Design review of the part built by this model. Coordinates are the model's own, in mm. A direction names the side the tool comes from. Give positions to 0.01 mm unless a question says otherwise; leave off trailing zeros. Order: outer loops, then holes, each group sorted by start corner. A loop starts at its lowest first (then second) coordinate and runs counter-clockwise, first axis right, second up. Notation, with made-up numbers: M -22.75,34 L -13.75,34 A36 ccw -13.75,70 Z; hole C -17.5,9 d4. An arc over 180 degrees is marked long. Answer as a JSON object with one key per item and string values.
Autodesk Inventor part; units mm, degrees
ref_plane "Work Plane1" through (1.525, 0, 0) normal (0, 0, 1) x (1, 0, 0)
ref_plane "YZ Plane" through (0, 0, 0) normal (1, 0, 0) x (0, 1, 0)
ref_plane "XZ Plane" through (0, 0, 0) normal (0, 1, 0) x (-1, 0, 0)
sketch "Sketch1" plane through (0, 0, 0) normal (0, 0, 1) x (1, 0, 0)
  line L0 (0, 5.0006) -> (0, 3.175)
  line L1 (3.175, 3.175) -> (22.225, 3.175)
  line L2 (22.225, 3.175) -> (22.225, 0)
  line L3 (22.225, 0) -> (-0.6351, 0)
  line L4 (-5.2071, 0) -> (26.797, 0)
  line L5 (-0.6351, 0) -> (-0.6351, 5.0006)
  line L6 (-0.6351, 5.0006) -> (0, 5.0006)
  line L7 (3.175, 3.175) -> (1.9049, 3.175)
  line L8 (1.9049, 3.175) -> (0, 3.175)
  line L9 (0, -1.0001) -> (0, 6.0007)
  dimension "d0" = 22.225
  dimension "d1" = 19.05
  dimension "d2" = 6.35
  dimension "d9" = 0.6351
  dimension "d10" = 10.0013
  dimension "d13" = 1.2701
  dimension "d14" = 6.35
revolve "Body" add sketch "Sketch1" angle 360 about axis through (22.225, 0, 0) along (-1, 0, 0)
sketch "Sketch2" plane through (-0.6351, 0, 0) normal (-1, 0, 0) x (0, 0, 1)
  line L0 (0, 6.4158) -> (5.5562, 3.2079)
  line L1 (5.5562, 3.2079) -> (5.5562, -3.2079)
  line L2 (5.5562, -3.2079) -> (0, -6.4158)
  line L3 (0, -6.4158) -> (-5.5562, -3.2079)
  line L4 (-5.5562, -3.2079) -> (-5.5562, 3.2079)
  line L5 (-5.5562, 3.2079) -> (0, 6.4158)
  point P0 (0, 0)
  point P1 (0, 0)
  dimension "d11" = 11.1125
extrude "Head" add sketch "Sketch2" along normal blind 3.3337
sketch "Sketch4" plane through (0, 0, 0) normal (0, 0, 1) x (1, 0, 0)
  line L0 (-3.9689, 5.5563) -> (-3.9689, 6.4158)
  line L1 (-3.9689, 6.4158) -> (-3.4726, 6.4158)
  line L2 (-3.4726, 6.4158) -> (-3.9689, 5.5563)
  line L3 (-4.6356, 0) -> (0.0317, 0)
  line L4 (-0.6351, 6.4158) -> (-3.9688, 6.4158)
  line L5 (-3.9688, 3.2079) -> (-3.9688, 6.4158)
  dimension "d5" = 30
  dimension "d19" = 11.1125
revolve "Chamfer1" cut sketch "Sketch4" angle 360 about axis through (-10, 0, 0) along (1, 0, 0)
thread "Thread"
chamfer "Chamfer2" distance 0.6875 distance2 1.2701 1 edges at (22.225, -3.175, 0) measured on face at (22.225, -0.1276, -1.0506)
ref_plane "Work Plane1" through (1.525, 0, 0) normal (0, 0, 1) x (1, 0, 0)
fillet "Fillet2" radius 0.635 1 edges at (0, -3.175, 0)
equation "\"d0\" = NLG"
equation "\"d1\" = GEL"
equation "\"d2\" = GD"
equation "\"d10\" = SD2"
equation "\"d14\" = BDM"
equation "\"d11\" = SW"
equation "\"d3\" = KOH - SD"
equation "\"d5\" = ANG1"
equation "\"d19\" = SW0"
equation "\"d63\" = R"
equation "\"d15\" = GEL"
equation "\"d6\" = -0.5 * SPD + 0.5 * GD"
equation "\"NLG\" = 22.225"
equation "\"GD\" = NND"
equation "\"BDM\" = 6.35"
equation "\"KOH\" = 3.96875"
equation "\"GEL\" = 19.05"
equation "\"SW\" = 11.1125"
equation "\"SW0\" = SW"
equation "\"SPD\" = 4.9751"
equation "\"SD2\" = 10.00125"
equation "\"SD\" = 0.635"
equation "\"ANG1\" = 30deg"
equation "\"GAL\" = 1.27"
equation "\"GUL\" = 1.27"
equation "\"R\" = 0.635"
equation "\"d62\" = -NLG - SD + GUL"
equation "\"THREADDIA\" = 6.35"
equation "\"TOA\" = 30deg"
equation "\"RR\" = 0.254"
equation "\"NND\" = 6.35"
equation "\"E0\" = 1.155 * SW"
equation "\"SLG\" = 0"
equation "\"GD1\" = 4.9751"
properties part number "ANSI B18.2.1 - 1/4-20 UNC - 0.875" material "Steel, Mild"
(1) We need section A-A (x = 15.75). Write out the cut boundary in (y, z) (3 decimals).
Checked values:
{"outline": "C 0,0 d6.35"}
(2) To check wall thickness, follow L1, parallel to X at y = 1.25, z = 4.25; L2, parallel to X at y = 5.75, z = 1; L3, parallel to Z at x = 4.5, y = -2.75. State the ranges of each line that lie inside material, in increasing order. Write a range as from..to.
Checked values:
{"L1": "x = -3.97..0", "L2": "x = -3.81..-0.64", "L3": "z = -1.59..1.59"}
(3) Insertion check: pin 1 (5 mm diameter, centred on x = 12.5, z = 4.5, fed in from -Y); pin 2 (3 mm diameter, centred on x = 9, y = -2.5, fed in from -Z); pin 3 (2 mm diameter, centred on y = -3.5, z = -0.5, fed in from +X). Each pin has a flat end and moves straight along its axis. Give the tip position at first contact, or say it passes through.
Checked values:
{"pin 1": "stops at y = -2.47", "pin 2": "stops at z = -3.01", "pin 3": "stops at x = 22.14"}
(4) Tool access review of faces 1 (the flat face through (0, -1, 4)), 2 (the flat face through (-2.279, -4.834, -2.739)): name each direction out of +Z, -Z, +X, -X, +Y, -Y from which nothing blocks a thin tool from reaching the whole face with its end or side.
Checked values:
{"face 1": "+X", "face 2": "-Z, +X, -X, -Y"}
